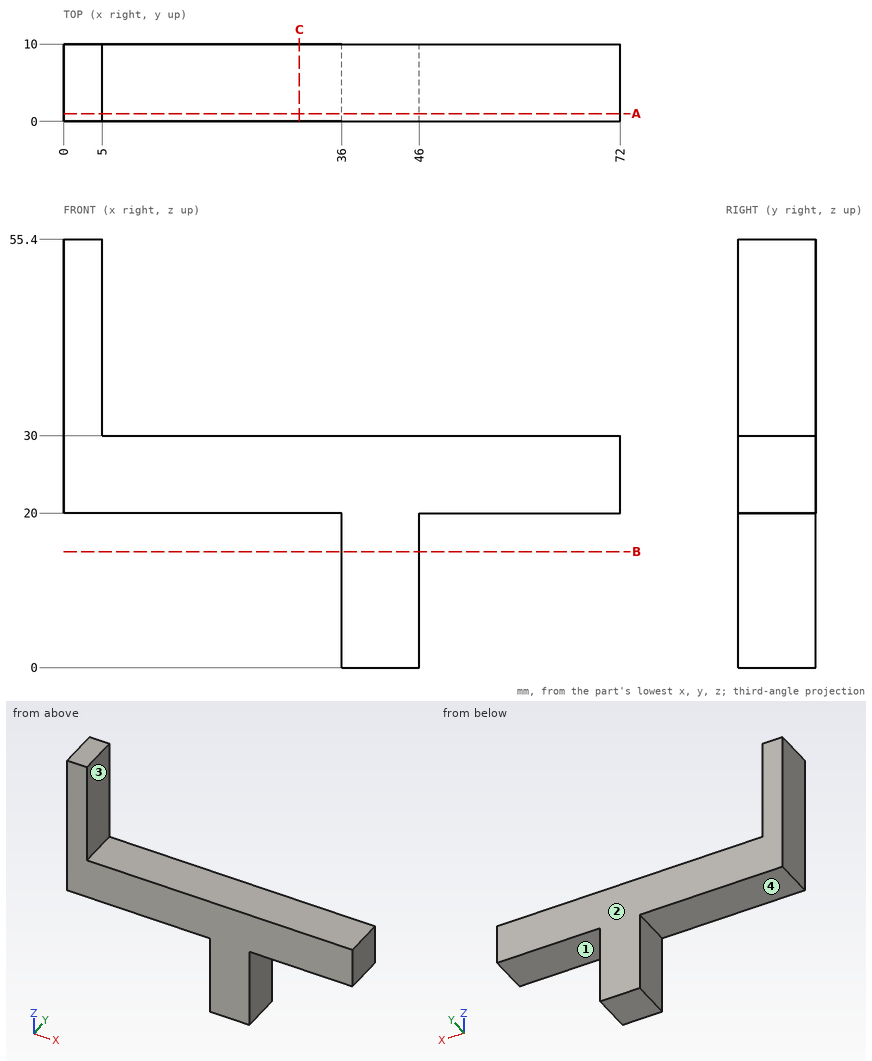
For this review, use the dimensioned drawing (mm, ordinates from the lowest corner) and the shaded views. A direction names the side the tool comes from. Give positions to 0.01 mm unless a question says otherwise; leave off trailing zeros. Loops run counter-clockwise (first coordinate to the right, second up) from the corner with the lowest first, then second, coordinate; pieces in that order, holes last. Notation, with made-up numbers: (79, 42.5) -> (89, 42.5) arc R12 ccw to (89, 54.5) -> close; hole circle Ø11 at (49.5, 39.25). An arc over 180 degrees is marked (long way). Use CSV: the item, a comma, the result in double quotes.
1. To check wall thickness, follow probe 1 along X at (y, z) = (6.75, 32); probe 2 along Z at (x, y) = (51.5, 1.75); probe 3 along X at (y, z) = (2.5, 13.5). State the ranges of each line that lie inside material, in increasing order. Write a range as from..to.
Result:
probe 1,"x = 0..5"
probe 2,"z = 20..30"
probe 3,"x = 36..46"
2. Machinability: for the marked faces 1, 2, 3 and 4, which of the approach directions +Z, -Z, +X, -X, +Y, -Y give a long, thin tool a straight path to every point of the face, cutting with its end or side? Answer none if there is none.
Result:
face 1,"-Z, +X, +Y, -Y"
face 2,"+Z, -Z, +X, -X, +Y"
face 3,"+Z, +X, +Y, -Y"
face 4,"-Z, -X, +Y, -Y"
3. For P1, Ø1.5, axis at x = 14, y = 2.5, coming from the -Z side; P2, Ø5, axis at x = 33.5, y = 6, coming from the +Z side; P3, Ø1, axis at y = 3, z = 46, coming from the +X side, all flat-tipped, find the tip position at first contact; note any pin that passes through.
Result:
P1,"stops at z = 20"
P2,"stops at z = 30"
P3,"stops at x = 5"
4. Consider section B-B, the plane z = 15. Write out the cut boundary in (x, y), then the cut area to 3 significant figures.
Result:
outline,"(36, 0) -> (46, 0) -> (46, 10) -> (36, 10) -> close"
area,"100 mm²"
5. Consider section C-C, the plane x = 30.5. Write out the cut boundary in (y, z), then the cut area to 3 significant figures.
Result:
outline,"(0, 20) -> (10, 20) -> (10, 30) -> (0, 30) -> close"
area,"100 mm²"
6. Consider section A-A, the plane y = 1. Write out the cut boundary in (x, z).
Result:
outline,"(0, 20) -> (36, 20) -> (36, 0) -> (46, 0) -> (46, 20) -> (72, 20) -> (72, 30) -> (5, 30) -> (5, 55.4) -> (0, 55.4) -> close"
